Here's how the part is built. I have some questions about the finished solid (model axes, mm). A direction names the side the tool comes from. Round coordinates to 2 decimals unless told otherwise and drop trailing zeros. Write each loop counter-clockwise with the first axis right and the second up, starting at its lowest first coordinate (ties: lowest second). Pieces come first, ordered by that corner, then holes. Notation, with made-up numbers: (85, 59.5) -> (112, 59.5) arc R16 ccw to (112, 63.5) -> close; hole circle Ø11 at (33, 58.25). An arc over 180 degrees is marked (long way). Answer in a Markdown table with one row per item. Add a question column.
from build123d import *

# Parameters (mm, degrees)
SKETCH_1_R               = 1.4
SKETCH_1_R_2             = 2
EXTRUDE_1_DEPTH          = 4
FILLET_1_R               = 66
CUT_EXTRUDE_1_DEPTH      = 145.092986744
CUT_EXTRUDE_1_DEPTH_BACK = 145.092986744
SKETCH_2_W               = 17.6
SKETCH_2_H               = 11.1
FILLET_3_R               = 0.5


with BuildPart() as part:
    # 草图1 → 凸台-拉伸1 (new body)
    with BuildSketch(Plane.XY):
        with BuildLine():
            Line((-97.873903688, 10.8), (-85.873903688, 10.8))
            ThreePointArc((-85.873903688, 10.8), (-83.8940047, 9.979898987), (-83.073903688, 8))
            ThreePointArc((-83.073903688, 8), (-83.1796222, 7.237866637), (-83.48879459, 6.53328442))
            Line((-83.48879459, 6.53328442), (-84.431683177, 5))
            ThreePointArc((-84.431683177, 5), (-84.652520599, 4.496726988), (-84.728033822, 3.952346014))
            Line((-84.728033822, 3.952346014), (-84.728033822, -3.047653986))
            ThreePointArc((-84.728033822, -3.047653986), (-84.969263339, -4.415734559), (-85.66385605, -5.618804425))
            Line((-85.66385605, -5.618804425), (-99.33833884, -21.915418417))
            Line((-99.33833884, -21.915418417), (-113.429667528, -58.624584688))
            ThreePointArc((-113.429667528, -58.624584688), (-113.541543089, -61.69465347), (-111.747141559, -64.18823756))
            ThreePointArc((-111.747141559, -64.18823756), (-108.724804348, -68.153933924), (-108.495917327, -73.134785316))
            ThreePointArc((-108.495917327, -73.134785316), (-109.387053216, -74.479515508), (-110.913984241, -75))
            Line((-110.913984241, -75), (-116.470682802, -75))
            ThreePointArc((-116.470682802, -75), (-121.827503028, -72.18164054), (-122.538955574, -66.170608328))
            Line((-122.538955574, -66.170608328), (-99.683969288, -6.631333481))
            ThreePointArc((-99.683969288, -6.631333481), (-99.187224477, -4.870009241), (-99.019773553, -3.047653986))
            Line((-99.019773553, -3.047653986), (-99.019773553, 3.952346014))
            ThreePointArc((-99.019773553, 3.952346014), (-99.095286776, 4.496726988), (-99.316124198, 5))
            Line((-99.316124198, 5), (-100.259012785, 6.53328442))
            ThreePointArc((-100.259012785, 6.53328442), (-100.568185176, 7.237866637), (-100.673903688, 8))
            ThreePointArc((-100.673903688, 8), (-99.853802675, 9.979898987), (-97.873903688, 10.8))
        make_face()
        with Locations((-85.873903688, 8)):
            Circle(SKETCH_1_R, mode=Mode.SUBTRACT)
        with Locations((-97.873903688, 8)):
            Circle(SKETCH_1_R, mode=Mode.SUBTRACT)
        with Locations((-97.673903688, -14.1)):
            Circle(SKETCH_1_R, mode=Mode.SUBTRACT)
        with Locations((-91.873903688, -5.1)):
            Circle(SKETCH_1_R, mode=Mode.SUBTRACT)
        with Locations((-115.399537808, -68.5)):
            Circle(SKETCH_1_R_2, mode=Mode.SUBTRACT)
        with BuildLine():
            Line((-88.763801636, 5.1), (-94.984005739, 5.1))
            ThreePointArc((-94.984005739, 5.1), (-95.172987976, 5.13708995), (-95.333932845, 5.242857143))
            ThreePointArc((-95.333932845, 5.242857143), (-95.615325044, 5.241421356), (-95.61676083, 4.960029158))
            ThreePointArc((-95.61676083, 4.960029158), (-95.510993638, 4.799084288), (-95.473903688, 4.610102051))
            Line((-95.473903688, 4.610102051), (-95.473903688, 0.389897949))
            ThreePointArc((-95.473903688, 0.389897949), (-95.510993638, 0.200915712), (-95.61676083, 0.039970842))
            ThreePointArc((-95.61676083, 0.039970842), (-95.615325044, -0.241421356), (-95.333932845, -0.242857143))
            ThreePointArc((-95.333932845, -0.242857143), (-95.172987976, -0.13708995), (-94.984005739, -0.1))
            Line((-94.984005739, -0.1), (-88.763801636, -0.1))
            ThreePointArc((-88.763801636, -0.1), (-88.5748194, -0.13708995), (-88.41387453, -0.242857143))
            ThreePointArc((-88.41387453, -0.242857143), (-88.132482331, -0.241421356), (-88.131046545, 0.039970842))
            ThreePointArc((-88.131046545, 0.039970842), (-88.236813737, 0.200915712), (-88.273903688, 0.389897949))
            Line((-88.273903688, 0.389897949), (-88.273903688, 4.610102051))
            ThreePointArc((-88.273903688, 4.610102051), (-88.236813737, 4.799084288), (-88.131046545, 4.960029158))
            ThreePointArc((-88.131046545, 4.960029158), (-88.132482331, 5.241421356), (-88.41387453, 5.242857143))
            ThreePointArc((-88.41387453, 5.242857143), (-88.5748194, 5.13708995), (-88.763801636, 5.1))
        make_face(mode=Mode.SUBTRACT)
    extrude(amount=EXTRUDE_1_DEPTH)

    # 圆角1
    fillet_1_edges = [part.edges().sort_by_distance(p)[0] for p in [
        (-99.33833884, -21.915418417, 2),
    ]]
    fillet(fillet_1_edges, radius=FILLET_1_R)

    # 草图2 → 切除-拉伸1 (cut, two sides: drawn at the far end of the back side and taken through both)
    with BuildSketch(Plane.XY.offset(4).offset(-CUT_EXTRUDE_1_DEPTH_BACK)):
        with Locations((-91.873903688, 5.25)):
            Rectangle(SKETCH_2_W, SKETCH_2_H)
    extrude(amount=CUT_EXTRUDE_1_DEPTH + CUT_EXTRUDE_1_DEPTH_BACK, mode=Mode.SUBTRACT)

    # 圆角3
    fillet_3_edges = [part.edges().sort_by_distance(p)[0] for p in [
        (-99.019773553, -0.3, 2),
        (-84.728033822, -0.3, 2),
    ]]
    fillet(fillet_3_edges, radius=FILLET_3_R)


solid = part.part
Item 1: On a 3-axis mill with a long thin cutter (end or side, diameter ignored), from which of +Z, -Z, +X, -X, +Y, -Y can I reach the whole of each face in a straight line? I mean faces 1 (the flat face through (-108.29, -45.24, 1.97)), 2 (the flat face through (-99.02, -2, 2)), 3 (the flat face through (-105, -35, 0)). Say none if no direction works.
Item 2: If we mould it in two halves opening along Y, with no side actions, what happens to faces 4 (the cylindrical face through (-116.874, -67.148, 1.972)), 5 (the cylindrical face through (-121.78, -72.25, 1.97)), 6 (the cylindrical face through (-96.34, -13.68, 1.97)), 7 (the flat face through (-111.271, -36.818, 1.972))? For each: pulls with the +Y half, pulls with the -Y half, needs draft (parallel to the pull), parting line crosses it, or undercut.
Item 3: If we section it at B-B on x = -114.5: Please give me the cut outline in (y, z).
Item 4: If we section it at D-D on y = -19: Please give me the cut outline in (x, z), then the cut area to 3 significant figures.
Item 5: If we section it at A-A on z = 1.35: Please give me the cut outline in (x, y).
Item 6: I need wall thicknesses on line 1 along Y through (x, z) = (-91, 2.15); line 2 along Y through (x, z) = (-97, 2.7); line 3 along X through (y, z) = (-58.5, 0.25). Which ranges of each line are inside material? Lowest first, please. Write a range as from..to.
Item 7: If we section it at C-C on y = -68.5: Please give me the cut outline in (x, z), then the cut area to 3 significant figures.
Results list:
| question | item | result |
|---|---|---|
| 1 | face 1 | +Z, -Z, +X |
| 1 | face 2 | +Z, -Z, -X, +Y |
| 1 | face 3 | -Z, +X, -X, +Y, -Y |
| 2 | face 4 | undercut |
| 2 | face 5 | parting line crosses it |
| 2 | face 6 | undercut |
| 2 | face 7 | pulls with the +Y half |
| 3 | outline | (-75, 0) -> (-70.29, 0) -> (-70.29, 4) -> (-75, 4) -> close; (-66.71, 0) -> (-45.23, 0) -> (-45.23, 4) -> (-66.71, 4) -> close |
| 4 | outline | (-104.43, 0) -> (-96.42, 0) -> (-96.42, 4) -> (-104.43, 4) -> close |
| 4 | area | 32.1 mm² |
| 5 | outline | (-122.54, -66.17) arc R6.5 ccw to (-116.47, -75) -> (-110.91, -75) arc R2.5 ccw to (-108.5, -73.13) arc R8.36 ccw to (-111.75, -64.19) arc R4.74 cw to (-113.43, -58.62) -> (-103.3, -32.23) arc R66 cw to (-92.24, -13.45) -> (-85.66, -5.62) arc R4 ccw to (-84.73, -3.05) -> (-84.73, -0.8) arc R0.5 ccw to (-85.23, -0.3) -> (-98.52, -0.3) arc R0.5 ccw to (-99.02, -0.8) -> (-99.02, -3.05) arc R10 cw to (-99.68, -6.63) -> close; hole circle Ø4 at (-115.4, -68.5); hole circle Ø2.8 at (-97.67, -14.1); hole circle Ø2.8 at (-91.87, -5.1) |
| 6 | line 1 | -11.98..-6.19, -4.01..-0.3 |
| 6 | line 2 | -19.88..-15.33, -12.87..-0.3 |
| 6 | line 3 | -119.59..-113.38 |
| 7 | outline | (-122.97, 0) -> (-117.4, 0) -> (-117.4, 4) -> (-122.97, 4) -> close; (-113.4, 0) -> (-108.61, 0) -> (-108.61, 4) -> (-113.4, 4) -> close |
| 7 | area | 41.5 mm² |
